from build123d import *

# Parameters (mm, degrees)
F0_W     = 24
F0_H     = 240
F1_DEPTH = 9
F2_W     = 9
F2_H     = 12
F3_DEPTH = 9
F4_W     = 12
F4_H     = 9
F4_W_2   = 2
F5_DEPTH = 9


with BuildPart() as f1:
    # F0 (on Right) → F1 (new body)
    with BuildSketch(Plane.YZ):
        Rectangle(F0_W, F0_H)
    extrude(amount=F1_DEPTH)

    # F2 (on face) → F3 (join, through all)
    with BuildSketch(Plane.YZ.offset(9)):
        with Locations((-16.5, -114)):
            Rectangle(F2_W, F2_H)
        with Locations((-16.5, -90)):
            Rectangle(F2_W, F2_H)
        with Locations((-16.5, -66)):
            Rectangle(F2_W, F2_H)
        with Locations((-16.5, -42)):
            Rectangle(F2_W, F2_H)
        with Locations((-16.5, -18)):
            Rectangle(F2_W, F2_H)
        with Locations((-16.5, 6)):
            Rectangle(F2_W, F2_H)
        with Locations((-16.5, 30)):
            Rectangle(F2_W, F2_H)
        with Locations((-16.5, 54)):
            Rectangle(F2_W, F2_H)
        with Locations((-16.5, 78)):
            Rectangle(F2_W, F2_H)
        with Locations((-16.5, 102)):
            Rectangle(F2_W, F2_H)
        with Locations((16.5, -90)):
            Rectangle(F2_W, F2_H)
        with Locations((16.5, 30)):
            Rectangle(F2_W, F2_H)
        with Locations((16.5, 102)):
            Rectangle(F2_W, F2_H)
        with Locations((16.5, -18)):
            Rectangle(F2_W, F2_H)
        with Locations((16.5, 78)):
            Rectangle(F2_W, F2_H)
        with Locations((16.5, 6)):
            Rectangle(F2_W, F2_H)
        with Locations((16.5, 54)):
            Rectangle(F2_W, F2_H)
        with Locations((16.5, -42)):
            Rectangle(F2_W, F2_H)
        with Locations((16.5, -66)):
            Rectangle(F2_W, F2_H)
        with Locations((16.5, -114)):
            Rectangle(F2_W, F2_H)
    extrude(amount=-F3_DEPTH)

    # F4 (on face) → F5 (join, through all)
    with BuildSketch(Plane.YZ.offset(9)):
        with Locations((0, -124.5)):
            Rectangle(F4_W, F4_H)
        with Locations((20, -124.5)):
            Rectangle(F4_W_2, F4_H)
        with Locations((-20, -124.5)):
            Rectangle(F4_W_2, F4_H)
    extrude(amount=-F5_DEPTH)


solid = f1.part
Can you work these out from the model? Positions are in its coordinate system, mm. A direction names the side the tool comes from. Give positions to 0.01 mm unless a question says otherwise; leave off trailing zeros. Loops run counter-clockwise (first coordinate to the right, second up) from the corner with the lowest first, then second, coordinate; pieces in that order, holes last. Notation, with made-up numbers: (-25, -17.5) - (23, -17.5) arc R10 cw to (23, -1.5) - close; hole circle Ø10 at (-0.5, 44.25). An arc over 180 degrees is marked (long way). Return JSON: item names as keys, results as strings.
1. I want a section at A-A on z = 90. Please give me the cut outline in (x, y), and give its area (3 significant figures).
Output values:
{"outline": "(0, -12) - (9, -12) - (9, 12) - (0, 12) - close", "area": "216 mm²"}
2. If I drill on line 1 (Y direction, x = 1.75, z = -104); line 2 (Z direction, x = 2.5, y = -11), over which ranges is the centre line in solid material (lowest first)?
Output values:
{"line 1": "y = -12 to 12", "line 2": "z = -120 to 120"}
3. For faces 4 (the face through (5, 21, -42)), 5 (the face through (5, 16, 96)), 6 (the face through (5, -17, -96)), which set-ups out of +Z, -Z, +X, -X, +Y, -Y let a thin tool reach every point of the face, with its end or its side?
Output values:
{"face 4": "+Z, -Z, +X, -X, +Y", "face 5": "+X, -X, +Y", "face 6": "+X, -X, -Y"}
4. I'm going to push flat-ended pins straight in: pin 1 Ø2.5 at (x, z) = (5, 113.5) entering from -Y; pin 2 Ø2.5 at (x, y) = (5.5, 14.5) entering from +Z; pin 3 Ø1 at (y, z) = (-16, 23) entering from -X (1 decimal). Where does each tip first touch, or does it pass through?
Output values:
{"pin 1": "stops at y = -12", "pin 2": "stops at z = 108", "pin 3": "passes through"}
5. We'd pull the mould along Z, two halves only. Please class faces 1 (the face through (5, -17, 108)), 2 (the face through (5, -21, 102)), 3 (the face through (4, -12, -6)): +Z half, -Z half, draft (parallel to the pull), parting line (faces both ways), or undercut.
Output values:
{"face 1": "+Z half", "face 2": "draft", "face 3": "undercut"}
